Geometry check sheet. Reference: the model listing, model coordinates, mm. Face numbers are marked on the shaded views. A direction names the side the tool comes from. Round coordinates to 2 decimals unless told otherwise and drop trailing zeros. Order: outer loops, then holes, each group sorted by start corner. A loop starts at its lowest first (then second) coordinate and runs counter-clockwise, first axis right, second up. Notation, with made-up numbers: (61, 45) - (104, 45) arc R32 ccw to (104, 80) - close; hole circle Ø8 at (65.25, 75). An arc over 180 degrees is marked (long way). Use a Markdown table: item, result. Add a question column.
(1) Section check A-A on x = 2. Record the boundary of the cut face in (y, z) (3 decimals).
(2) Mould release check, pull along X, two halves, no side actions. Record for the marked faces 1, 2 and 3: released by +X, released by -X, zero draft, split by the parting line, or undercut.
(3) Section check D-D on y = -5. Record the boundary of the cut face in (x, z) (3 decimals), then the cut area to 3 significant figures.
(4) Access from +Z, -Z, +X, -X, +Y, -Y to the whole of each face (thin tool, end or side, straight path). Record for the marked faces 4 and 5.
(5) Gauge pin test, flat ends, axial feed: P1, Ø8, axis at y = -15.5, z = -29.5, coming from the -X side; P2, Ø1.5, axis at x = -17, z = 2, coming from the -Y side; P3, Ø1, axis at y = -26, z = 6, coming from the +X side. Record the tip position at first contact, or that the pin passes through.
(6) Thickness scan on line 1 along X through (y, z) = (-18, 2) (3 decimals); line 2 along Z through (x, y) = (-15, -2) (3 decimals); line 3 along Z through (x, y) = (-32, -5.25) (3 decimals). Record the ranges inside material, lowest first. Write a range as [from, to].
(7) Section check C-C on y = -21.5. Record the boundary of the cut face in (x, z) (3 decimals).
```python
from build123d import *

# Parameters (mm, degrees)
F1_DEPTH       = 6.35
F2_W           = 26.416
F2_H           = 3.175
F3_DEPTH       = 22.225
F4_W           = 3.175
F4_H           = 19.05
F5_DEPTH       = 8.255
F6_W           = 3.175
F6_H           = 3.175
F7_DEPTH       = 9.525
F8_W           = 3.175
F8_H           = 3.175
F9_DEPTH       = 9.525
F10_W          = 28.575
F10_H          = 3.175
F11_DEPTH      = 13.462
F12_W          = 3.175
F12_H          = 28.575
F13_DEPTH      = 50.8
F13_DEPTH_BACK = 3.175
F15_DEPTH      = 2.794
F17_DEPTH      = 25.4
F18_W          = 3.175
F18_H          = 3.175
F19_DEPTH      = 5.08
F20_W          = 28.575
F20_H          = 3.175
F21_DEPTH      = 6.35
F22_W          = 3.175
F22_H          = 3.175
F23_DEPTH      = 5.08


with BuildPart() as f1:
    # F0 (on Front) → F1 (new body)
    with BuildSketch(Plane.XZ):
        Polygon((0, 2.54), (0, 0), (3.175, 0), (6.35, 0), (6.35, 5.08), (6.35, 8.255), (-20.066, 8.255), (-20.066, 5.08), (-20.066, 0), (-16.891, 0), (-13.716, 0), (-13.716, 2.54), (-16.891, 2.54), (-16.891, 5.08), (3.175, 5.08), (3.175, 2.54), align=None)
    extrude(amount=F1_DEPTH)

    # F2 (on face) → F3 (join)
    with BuildSketch(Plane.XZ.offset(6.35)):
        with Locations((-6.858, 6.6675)):
            Rectangle(F2_W, F2_H)
    extrude(amount=F3_DEPTH)

    # F4 (on face) → F5 (join, through all)
    with BuildSketch(Plane.XY.offset(8.255)):
        with Locations((-21.6535, -9.525)):
            Rectangle(F4_W, F4_H)
        with Locations((7.9375, -9.525)):
            Rectangle(F4_W, F4_H)
    extrude(amount=-F5_DEPTH)

    # F6 (on face) → F7 (join, through all)
    with BuildSketch(Plane.XZ.offset(19.05)):
        with Locations((-21.6535, 1.5875)):
            Rectangle(F6_W, F6_H)
    extrude(amount=F7_DEPTH)

    # F8 (on face) → F9 (join, through all)
    with BuildSketch(Plane.XZ.offset(19.05)):
        with Locations((7.9375, 1.5875)):
            Rectangle(F8_W, F8_H)
    extrude(amount=F9_DEPTH)

    # F10 (on face) → F11 (join)
    with BuildSketch(Plane(origin=(-23.241, 0, 0), x_dir=(0, -1, 0), z_dir=(-1, 0, 0))):
        with Locations((14.2875, 1.5875)):
            Rectangle(F10_W, F10_H)
    extrude(amount=F11_DEPTH)

    # F12 (on face) → F13 (join, two sides)
    with BuildSketch(Plane(origin=(0, 0, 0), x_dir=(1, 0, 0), z_dir=(0, 0, -1))) as f13_sk:
        with Locations((-38.2905, 14.2875)):
            Rectangle(F12_W, F12_H)
    extrude(amount=F13_DEPTH)
    extrude(f13_sk.sketch, amount=-F13_DEPTH_BACK)

    # F14 (on face) → F15 (join)
    with BuildSketch(Plane(origin=(-39.878, 0, 0), x_dir=(0, -1, 0), z_dir=(-1, 0, 0))):
        Polygon((20.2565, 3.175), (14.2875, 3.175), (8.3185, 3.175), (8.3185, -21.463), (20.2565, -21.463), align=None)
    extrude(amount=F15_DEPTH)

    # F16 (on face) → F17 (cut)
    with BuildSketch(Plane.XY.offset(8.255)):
        with BuildLine():
            ThreePointArc((-10.361326316, -13.208), (-10.882090459, -11.9507641431), (-12.139326316, -11.43))
            Line((-12.139326316, -11.43), (-12.139326316, -13.208))
            Line((-12.139326316, -13.208), (-10.361326316, -13.208))
        make_face()
        with BuildLine():
            ThreePointArc((1.068673684, -13.208), (-0.709326316, -11.43), (-2.487326316, -13.208))
            ThreePointArc((-2.487326316, -13.208), (-0.709326316, -14.986), (1.068673684, -13.208))
        make_face()
        with BuildLine():
            Line((-12.139326316, -13.208), (-12.139326316, -11.43))
            ThreePointArc((-12.139326316, -11.43), (-13.3965621729, -14.4652358569), (-10.361326316, -13.208))
            Line((-10.361326316, -13.208), (-12.139326316, -13.208))
        make_face()
    extrude(amount=-F17_DEPTH, mode=Mode.SUBTRACT)

    # F18 (on face) → F19 (join, through all)
    with BuildSketch(Plane.XY.offset(3.175)):
        with Locations((-24.8285, -1.5875)):
            Rectangle(F18_W, F18_H)
    extrude(amount=F19_DEPTH)

    # F20 (on face) → F21 (join)
    with BuildSketch(Plane.YZ.offset(9.525)):
        with Locations((-14.2875, 1.5875)):
            Rectangle(F20_W, F20_H)
    extrude(amount=F21_DEPTH)

    # F22 (on face) → F23 (join, through all)
    with BuildSketch(Plane.XY.offset(3.175)):
        with Locations((11.1125, -1.5875)):
            Rectangle(F22_W, F22_H)
    extrude(amount=F23_DEPTH)


solid = f1.part
```
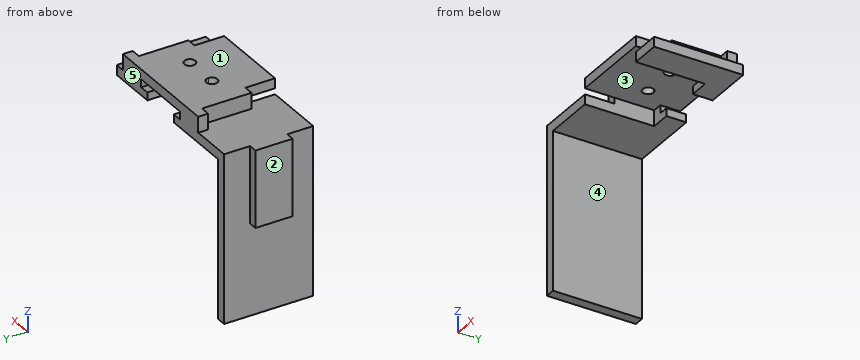
Check sheet entries:
| question | item | result |
|---|---|---|
| 1 | outline | (-28.575, 5.08) - (0, 5.08) - (0, 8.255) - (-28.575, 8.255) - close; (-6.35, 0) - (0, 0) - (0, 2.54) - (-6.35, 2.54) - close |
| 2 | face 1 | zero draft |
| 2 | face 2 | released by -X |
| 2 | face 3 | undercut |
| 3 | outline | (-39.878, -50.8) - (-36.703, -50.8) - (-36.703, 0) - (-13.716, 0) - (-13.716, 2.54) - (-16.891, 2.54) - (-16.891, 5.08) - (3.175, 5.08) - (3.175, 2.54) - (0, 2.54) - (0, 0) - (15.875, 0) - (15.875, 3.175) - (9.525, 3.175) - (9.525, 8.255) - (-23.241, 8.255) - (-23.241, 3.175) - (-39.878, 3.175) - close |
| 3 | area | 419 mm2 |
| 4 | face 4 | -Z, +X, +Y, -Y |
| 4 | face 5 | +Z, -Z, +X, -X, +Y |
| 5 | P1 | stops at x = -39.88 |
| 5 | P2 | stops at y = -6.35 |
| 5 | P3 | stops at x = 6.35 |
| 6 | line 1 | x = [-42.672, -20.066], [6.35, 15.875] |
| 6 | line 2 | z = [0, 2.54], [5.08, 8.255] |
| 6 | line 3 | z = [0, 3.175] |
| 7 | outline | (-39.878, -50.8) - (-36.703, -50.8) - (-36.703, 0) - (-20.066, 0) - (-20.066, 3.175) - (-39.878, 3.175) - close; (-20.066, 5.08) - (6.35, 5.08) - (6.35, 8.255) - (-20.066, 8.255) - close; (6.35, 0) - (15.875, 0) - (15.875, 3.175) - (6.35, 3.175) - close |
